For this review, take the finished solid that the model builds, in its own axes (mm). A direction names the side the tool comes from. Round coordinates to 2 decimals unless told otherwise and drop trailing zeros. Write each loop counter-clockwise with the first axis right and the second up, starting at its lowest first coordinate (ties: lowest second). Pieces come first, ordered by that corner, then holes. Notation, with made-up numbers: M 14,46 L 46,46 A14 ccw 46,73 Z; hole C -12,-13.5 d4. An arc over 180 degrees is marked long. Answer in a Markdown table with one row per item.
```python
from build123d import *

# Parameters (mm, degrees)
SKETCH_1_R                = 42.5
SKETCH_1_R_2              = 34
EXTRUDE_1_DEPTH           = 6
HOLE_WIZARD_1_D           = 3.6
HOLE_WIZARD_1_CBORE_D     = 6
HOLE_WIZARD_1_CBORE_DEPTH = 3.4
PATTERN_CIRCULAR_1_COUNT  = 12


with BuildPart() as part:
    # Sketch 1 → Extrude 1 (new body)
    with BuildSketch(Plane.XY):
        Circle(SKETCH_1_R)
        Circle(SKETCH_1_R_2, mode=Mode.SUBTRACT)
    extrude(amount=EXTRUDE_1_DEPTH)

    # Hole Wizard 1 (through all)
    with Locations(Plane(origin=(0, 0, 0), x_dir=(-1, 0, 0), z_dir=(0, 0, -1))):
        with Locations((0, 39)):
            hole_wizard_1 = CounterBoreHole(HOLE_WIZARD_1_D / 2, HOLE_WIZARD_1_CBORE_D / 2, HOLE_WIZARD_1_CBORE_DEPTH)

    # Pattern Circular 1: Hole Wizard 1 ×12 about axis
    pattern_circular_1_axis = Axis((0, 0, 0), (0, 0, 1))
    for i in range(1, PATTERN_CIRCULAR_1_COUNT):
        add(hole_wizard_1.rotate(pattern_circular_1_axis, i * 360 / PATTERN_CIRCULAR_1_COUNT), mode=Mode.SUBTRACT)


solid = part.part
```
Q1. Take a section at D-D (x = -25.5). State the section outline as (y, z) points, then the cut area to 3 significant figures.
Found:
| item | result |
|---|---|
| outline | M -34,0 L -22.49,0 L -22.49,6 L -34,6 Z; M 22.49,0 L 34,0 L 34,6 L 22.49,6 Z |
| area | 138 mm² |
Q2. Insertion check: P1, Ø4, axis at x = 33.77, y = -19.5, coming from the -Z side; P2, Ø1.5, axis at y = -6, z = 3, coming from the -X side; P3, Ø2, axis at x = -15, z = 5.5, coming from the +Y side. Each pin has a flat end and moves straight along its axis. Give the tip position at first contact, or say it passes through.
Found:
| item | result |
|---|---|
| P1 | z = 3.4 |
| P2 | x = -42.17 |
| P3 | y = 40.13 |
Q3. Take a section at B-B (y = 19.5). State the section outline as (x, z) points (3 decimals).
Found:
| item | result |
|---|---|
| outline | M -37.762,0 L -36.775,0 L -36.775,3.4 L -35.575,3.4 L -35.575,6 L -37.762,6 Z; M -31.975,3.4 L -30.775,3.4 L -30.775,0 L -27.852,0 L -27.852,6 L -31.975,6 Z; M 27.852,0 L 30.775,0 L 30.775,3.4 L 31.975,3.4 L 31.975,6 L 27.852,6 Z; M 35.575,3.4 L 36.775,3.4 L 36.775,0 L 37.762,0 L 37.762,6 L 35.575,6 Z |
Q4. Mouldability with a two-part tool opening along X and no side actions: class faces 3 (the face through (-33.727, -25.861, 2.958)), 4 (the face through (-19.421, 35.573, 4.718)), 5 (the face through (35.986, -17.472, 1.676)) as +X half, -X half, draft (parallel to the pull), parting line (faces both ways), or undercut.
Found:
| item | result |
|---|---|
| face 3 | parting line |
| face 4 | undercut |
| face 5 | undercut |
Q5. For probe 1 along Y at (x, z) = (0, 5.05); probe 2 along X at (y, z) = (-22, 1.45); probe 3 along X at (y, z) = (-36.5, 0.9), list the stretches that pass through material, from the lowest coordinate up.
Found:
| item | result |
|---|---|
| probe 1 | -42.5 to -40.8, -37.2 to -34, 34 to 37.2, 40.8 to 42.5 |
| probe 2 | -36.36 to -35.43, -32.12 to -25.92, 25.92 to 32.12, 35.43 to 36.36 |
| probe 3 | -21.77 to -20.75, -18.25 to -1.66, 1.66 to 18.25, 20.75 to 21.77 |
Q6. Machinability: for faces 1 (the face through (0, 42, 2)), 2 (the face through (19.421, -35.573, 4.718)), which of the approach directions +Z, -Z, +X, -X, +Y, -Y give a long, thin tool a straight path to every point of the face, cutting with its end or side? Answer none if there is none.
Found:
| item | result |
|---|---|
| face 1 | -Z |
| face 2 | +Z, -Z |
Q7. Take a section at A-A (x = 0). State the section outline as (y, z) points, then the cut area to 3 significant figures.
Found:
| item | result |
|---|---|
| outline | M -42.5,0 L -42,0 L -42,3.4 L -40.8,3.4 L -40.8,6 L -42.5,6 Z; M -37.2,3.4 L -36,3.4 L -36,0 L -34,0 L -34,6 L -37.2,6 Z; M 34,0 L 36,0 L 36,3.4 L 37.2,3.4 L 37.2,6 L 34,6 Z; M 40.8,3.4 L 42,3.4 L 42,0 L 42.5,0 L 42.5,6 L 40.8,6 Z |
| area | 42.5 mm² |
Q8. Take a section at C-C (z = 4.9). State how many separate pieces and enclosed holes the cut face has, then the cut area to 3 significant figures.
Found:
| item | result |
|---|---|
| separate pieces | 1 |
| enclosed holes | 13 |
| area | 1,920 mm² |
